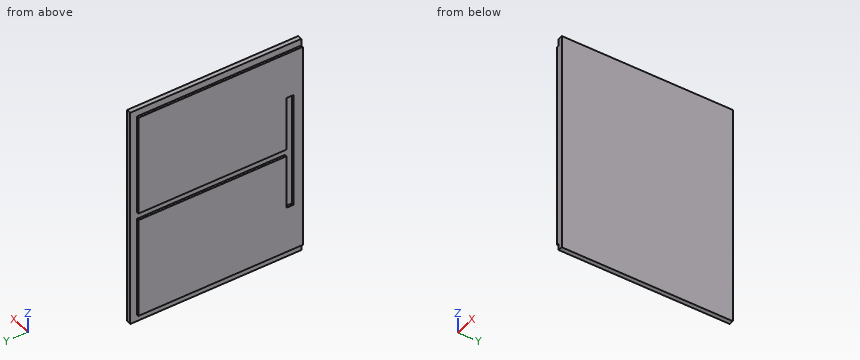
from build123d import *

# Parameters (mm, degrees)
F0_W     = 461.44942
F0_H     = 607.50196
F1_DEPTH = 18
F2_W     = 18
F2_H     = 19
F2_H_2   = 569.50196
F2_W_2   = 19
F2_H_3   = 315.40196
F3_DEPTH = 6
F4_W     = 416.292534
F4_H     = 19
F5_DEPTH = 6


with BuildPart() as f1:
    # F0 (on Right) → F1 (new body)
    with BuildSketch(Plane.YZ):
        with Locations((6.814488, 30.1922)):
            Rectangle(F0_W, F0_H)
    extrude(amount=F1_DEPTH)

    # F2 (on face) → F3 (cut)
    with BuildSketch(Plane(origin=(0, 0, 0), x_dir=(0, -1, 0), z_dir=(-1, 0, 0))):
        with Locations((-228.539198, 324.44318)):
            Rectangle(F2_W, F2_H)
        Polygon((180.510222, 333.94318), (-219.539198, 333.94318), (-219.539198, 314.94318), (223.910222, 314.94318), (223.910222, 333.94318), (198.510222, 333.94318), align=None)
        with Locations((-228.539198, 30.1922)):
            Rectangle(F2_W, F2_H_2)
        with Locations((-228.539198, -264.05878)):
            Rectangle(F2_W, F2_H)
        Polygon((223.910222, -254.55878), (-219.539198, -254.55878), (-219.539198, -273.55878), (180.510222, -273.55878), (198.510222, -273.55878), (223.910222, -273.55878), align=None)
        with Locations((189.010222, 30.1922)):
            Rectangle(F2_W_2, F2_H_3)
    extrude(amount=-F3_DEPTH, mode=Mode.SUBTRACT)

    # F4 (on face) → F5 (cut)
    with BuildSketch(Plane(origin=(0, 0, 0), x_dir=(0, -1, 0), z_dir=(-1, 0, 0))):
        with Locations((-18.287234, 30.1922)):
            Rectangle(F4_W, F4_H)
    extrude(amount=-F5_DEPTH, mode=Mode.SUBTRACT)


solid = f1.part
CAD build for the part. Positions are in the model's coordinates, mm. Round coordinates to 2 decimals unless told otherwise and drop trailing zeros. Loops run counter-clockwise (first coordinate to the right, second up) from the corner with the lowest first, then second, coordinate; pieces in that order, holes last.
(1) Cut at A-A (y = -24). Give the cut face in (x, z), plus the area to 3 significant figures.
(2) Drop flat-ended pins along their axis: pin 1 (1.8 mm diameter, centred on x = 2, y = 85, fed in from -Z); pin 2 (3 mm diameter, centred on x = 3.5, z = 147.5, fed in from +Y); pin 3 (1.8 mm diameter, centred on x = 3, y = -188.5, fed in from +Z). Give the stop position or say it passes through.
(3) Wall check: line 1 along Y through (x, z) = (3.75, 60.5); line 2 along Z through (x, y) = (1.75, 4.5); line 3 along Y through (x, z) = (2.25, 240). Give the ranges that are in metal, low to high.
(4) Cut at B-B (z = -30). Give the cut face in (x, y).
Findings below:
1. outline: (0, -254.56) - (6, -254.56) - (6, -273.56) - (18, -273.56) - (18, 333.94) - (6, 333.94) - (6, 314.94) - (0, 314.94) - (0, 39.69) - (6, 39.69) - (6, 20.69) - (0, 20.69) - close
1. area: 10,600 mm2
2. pin 1: stops at z = -254.56
2. pin 2: stops at y = 219.54
2. pin 3: stops at z = 314.94
3. line 1: y = -223.91 to -198.51, -179.51 to 219.54
3. line 2: z = -254.56 to 20.69, 39.69 to 314.94
3. line 3: y = -223.91 to 219.54
4. outline: (0, -223.91) - (18, -223.91) - (18, 237.54) - (6, 237.54) - (6, 219.54) - (0, 219.54) - (0, -179.51) - (6, -179.51) - (6, -198.51) - (0, -198.51) - close
